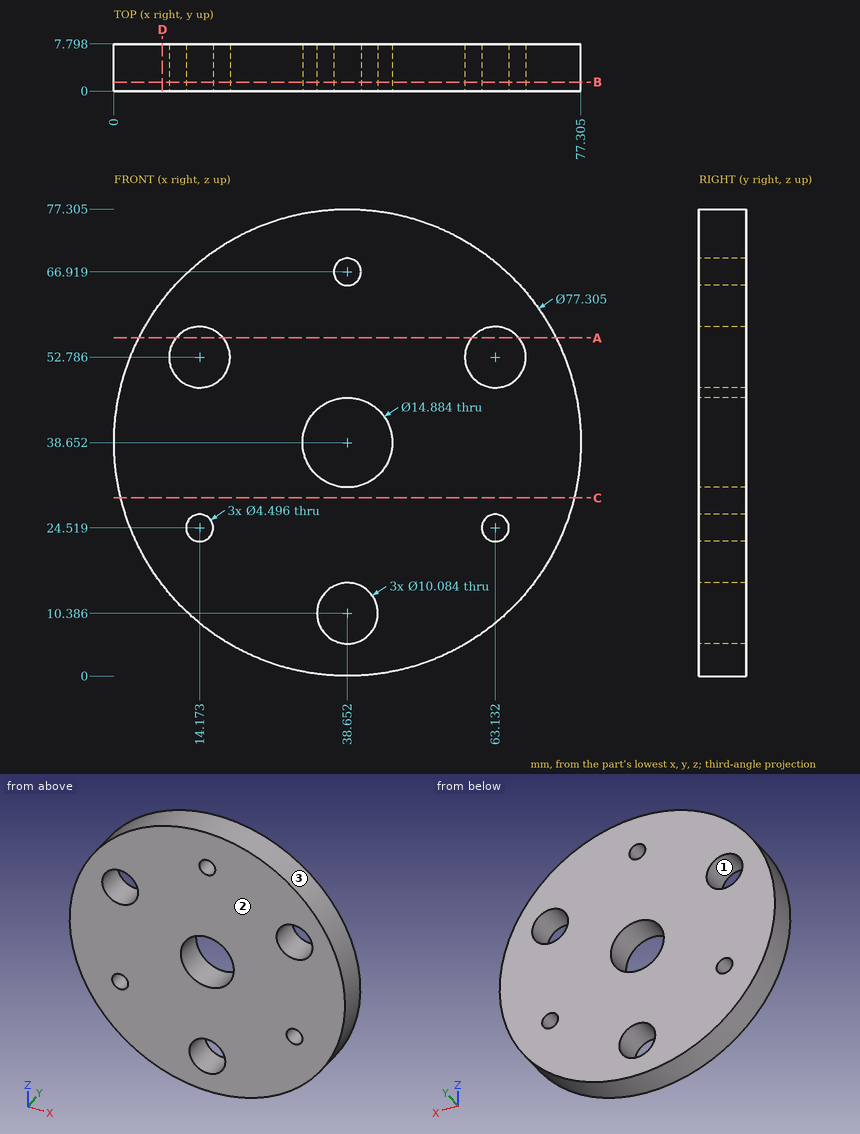
For this review, use the dimensioned drawing (mm, ordinates from the lowest corner) and the shaded views. Coordinates: 2 decimals unless noted, no trailing zeros. Write each loop counter-clockwise with the first axis right and the second up, starting at its lowest first coordinate (ties: lowest second). Pieces come first, ordered by that corner, then holes. Notation, with made-up numbers: (38, 81) -> (92, 81) arc R17 cw to (92, 89) -> close; hole circle Ø9 at (31, -23.5). An arc over 180 degrees is marked (long way). Put each result on its own line as item: value.
Q1. Take a section at A-A, the plane z = 56. State the section outline as (x, y) points.
From the geometry:
outline: (4.11, 0) -> (10.29, 0) -> (10.29, 7.8) -> (4.11, 7.8) -> close; (18.06, 0) -> (59.25, 0) -> (59.25, 7.8) -> (18.06, 7.8) -> close; (67.02, 0) -> (73.19, 0) -> (73.19, 7.8) -> (67.02, 7.8) -> close
Q2. Take a section at B-B, the plane y = 1.5. State the section outline as (x, z) points (1 decimal).
From the geometry:
outline: circle Ø77.3 at (38.7, 38.7); hole circle Ø10.1 at (14.2, 52.8); hole circle Ø4.5 at (14.2, 24.5); hole circle Ø14.9 at (38.7, 38.7); hole circle Ø10.1 at (38.7, 10.4); hole circle Ø4.5 at (38.7, 66.9); hole circle Ø10.1 at (63.1, 52.8); hole circle Ø4.5 at (63.1, 24.5)
Q3. Clearance check with flat-ended pins moving along their axes: pin 1 Ø4 at (x, y) = (21, 6.5) entering from -Z; pin 2 Ø13 at (x, z) = (63.13, 52.79) entering from +Y; pin 3 Ø2 at (y, z) = (2.5, 63.5) entering from -X (1 decimal). State where each tip first meets the part, or that it passes through.
From the geometry:
pin 1: stops at z = 3.31
pin 2: stops at y = 7.8
pin 3: stops at x = 8.2
Q4. The part is to be moulded in two halves that separate along X. For the marked faces 1, 2 and 3, say which applies: +X half, -X half, draft (parallel to the pull), parting line (faces both ways), or undercut.
From the geometry:
face 1: undercut
face 2: draft
face 3: parting line
Q5. Wall thickness on L1, parallel to X at y = 1.5, z = 55 (1 decimal); L2, parallel to X at y = 4.25, z = 53.5 (1 decimal); L3, parallel to Z at x = 14, y = 0.5 (1 decimal): over which ranges is each line inside the solid? List them lowest first.
From the geometry:
L1: x = 3.6 to 9.6, 18.7 to 58.6, 67.7 to 73.7
L2: x = 3 to 9.2, 19.2 to 58.1, 68.1 to 74.3
L3: z = 8.9 to 22.3, 26.8 to 47.7, 57.8 to 68.4
Q6. Take a section at C-C, the plane z = 29.5. State the section outline as (x, y) points (1 decimal).
From the geometry:
outline: (1.1, 0) -> (76.2, 0) -> (76.2, 7.8) -> (1.1, 7.8) -> close
Q7. Take a section at D-D, the plane x = 8. State the section outline as (y, z) points, then the cut area to 3 significant figures.
From the geometry:
outline: (0, 15.11) -> (7.8, 15.11) -> (7.8, 62.2) -> (0, 62.2) -> close
area: 367 mm2
